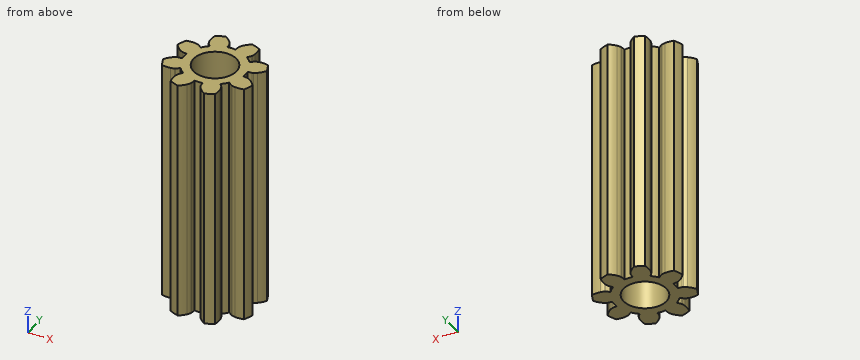
Autodesk Inventor part; units mm, degrees
ref_plane "YZ Plane" through (0, 0, 0) normal (1, 0, 0) x (0, 1, 0)
ref_plane "XZ Plane" through (0, 0, 0) normal (0, 1, 0) x (-1, 0, 0)
ref_plane "XY Plane" through (0, 0, 0) normal (0, 0, 1) x (1, 0, 0)
sketch "Sketch2" plane through (0, 0, 0) normal (0, 0, 1) x (1, 0, 0)
  arc A0 (0.2626, 1.917) -> (0.2462, 1.8632) centre (0.4994, 1.8157) ccw
  arc A1 (0.3627, 2.0876) -> (0.2626, 1.917) centre (0.9307, 1.6395) ccw
  arc A2 (0.7114, 2.3967) -> (0.3627, 2.0876) centre (1.3933, 1.2761) ccw
  arc A3 (-1.1698, 1.5411) -> (-1.1434, 1.4916) centre (-0.9308, 1.637) ccw
  arc A4 (-1.2197, 1.7326) -> (-1.1698, 1.5411) centre (-0.5012, 1.8175) ccw
  arc A5 (-1.1917, 2.1977) -> (-1.2197, 1.7326) centre (0.0829, 1.8876) ccw
  arc A6 (-1.917, 0.2626) -> (-1.8632, 0.2462) centre (-1.8157, 0.4994) ccw
  arc A7 (-2.0876, 0.3627) -> (-1.917, 0.2626) centre (-1.6395, 0.9307) ccw
  arc A8 (-2.3967, 0.7114) -> (-2.0876, 0.3627) centre (-1.2761, 1.3933) ccw
  arc A9 (-1.5411, -1.1698) -> (-1.4916, -1.1434) centre (-1.637, -0.9308) ccw
  arc A10 (-1.7326, -1.2197) -> (-1.5411, -1.1698) centre (-1.8175, -0.5012) ccw
  arc A11 (-2.1977, -1.1917) -> (-1.7326, -1.2197) centre (-1.8876, 0.0829) ccw
  arc A12 (-0.2626, -1.917) -> (-0.2462, -1.8632) centre (-0.4994, -1.8157) ccw
  arc A13 (-0.3627, -2.0876) -> (-0.2626, -1.917) centre (-0.9307, -1.6395) ccw
  arc A14 (-0.7114, -2.3967) -> (-0.3627, -2.0876) centre (-1.3933, -1.2761) ccw
  arc A15 (1.1698, -1.5411) -> (1.1434, -1.4916) centre (0.9308, -1.637) ccw
  arc A16 (1.2197, -1.7326) -> (1.1698, -1.5411) centre (0.5012, -1.8175) ccw
  arc A17 (1.1917, -2.1977) -> (1.2197, -1.7326) centre (-0.0829, -1.8876) ccw
  arc A18 (1.917, -0.2626) -> (1.8632, -0.2462) centre (1.8157, -0.4994) ccw
  arc A19 (2.0876, -0.3627) -> (1.917, -0.2626) centre (1.6395, -0.9307) ccw
  arc A20 (2.3967, -0.7114) -> (2.0876, -0.3627) centre (1.2761, -1.3933) ccw
  arc A21 (1.5411, 1.1698) -> (1.4916, 1.1434) centre (1.637, 0.9308) ccw
  arc A22 (1.7326, 1.2197) -> (1.5411, 1.1698) centre (1.8175, 0.5012) ccw
  arc A23 (2.1977, 1.1917) -> (1.7326, 1.2197) centre (1.8876, -0.0829) ccw
  arc A24 (-0.2462, 1.8632) -> (-0.2626, 1.917) centre (-0.4994, 1.8157) ccw
  arc A25 (-0.2626, 1.917) -> (-0.3627, 2.0876) centre (-0.9307, 1.6395) ccw
  arc A26 (-0.3627, 2.0876) -> (-0.7114, 2.3967) centre (-1.3933, 1.2761) ccw
  arc A27 (-1.4916, 1.1434) -> (-1.5411, 1.1698) centre (-1.637, 0.9308) ccw
  arc A28 (-1.5411, 1.1698) -> (-1.7326, 1.2197) centre (-1.8175, 0.5012) ccw
  arc A29 (-1.7326, 1.2197) -> (-2.1977, 1.1917) centre (-1.8876, -0.0829) ccw
  arc A30 (-1.8632, -0.2462) -> (-1.917, -0.2626) centre (-1.8157, -0.4994) ccw
  arc A31 (-1.917, -0.2626) -> (-2.0876, -0.3627) centre (-1.6395, -0.9307) ccw
  arc A32 (-2.0876, -0.3627) -> (-2.3967, -0.7114) centre (-1.2761, -1.3933) ccw
  arc A33 (-1.1434, -1.4916) -> (-1.1698, -1.5411) centre (-0.9308, -1.637) ccw
  arc A34 (-1.1698, -1.5411) -> (-1.2197, -1.7326) centre (-0.5012, -1.8175) ccw
  arc A35 (-1.2197, -1.7326) -> (-1.1917, -2.1977) centre (0.0829, -1.8876) ccw
  arc A36 (0.2462, -1.8632) -> (0.2626, -1.917) centre (0.4994, -1.8157) ccw
  arc A37 (0.2626, -1.917) -> (0.3627, -2.0876) centre (0.9307, -1.6395) ccw
  arc A38 (0.3627, -2.0876) -> (0.7114, -2.3967) centre (1.3933, -1.2761) ccw
  arc A39 (1.4916, -1.1434) -> (1.5411, -1.1698) centre (1.637, -0.9308) ccw
  arc A40 (1.5411, -1.1698) -> (1.7326, -1.2197) centre (1.8175, -0.5012) ccw
  arc A41 (1.7326, -1.2197) -> (2.1977, -1.1917) centre (1.8876, 0.0829) ccw
  arc A42 (1.8632, 0.2462) -> (1.917, 0.2626) centre (1.8157, 0.4994) ccw
  arc A43 (1.917, 0.2626) -> (2.0876, 0.3627) centre (1.6395, 0.9307) ccw
  arc A44 (2.0876, 0.3627) -> (2.3967, 0.7114) centre (1.2761, 1.3933) ccw
  arc A45 (1.1434, 1.4916) -> (1.1698, 1.5411) centre (0.9308, 1.637) ccw
  arc A46 (1.1698, 1.5411) -> (1.2197, 1.7326) centre (0.5012, 1.8175) ccw
  arc A47 (1.2197, 1.7326) -> (1.1917, 2.1977) centre (-0.0829, 1.8876) ccw
  arc A48 (0.2162, 1.6358) -> (-0.2162, 1.6358) centre (0, 0) ccw
  arc A49 (-1.0038, 1.3095) -> (-1.3095, 1.0038) centre (0, 0) ccw
  arc A50 (-1.6358, 0.2162) -> (-1.6358, -0.2162) centre (0, 0) ccw
  arc A51 (-1.3095, -1.0038) -> (-1.0038, -1.3095) centre (0, 0) ccw
  arc A52 (-0.2162, -1.6358) -> (0.2162, -1.6358) centre (0, 0) ccw
  arc A53 (1.0038, -1.3095) -> (1.3095, -1.0038) centre (0, 0) ccw
  arc A54 (1.6358, -0.2162) -> (1.6358, 0.2162) centre (0, 0) ccw
  arc A55 (1.3095, 1.0038) -> (1.0038, 1.3095) centre (0, 0) ccw
  arc A56 (-0.7114, 2.3967) -> (-1.1917, 2.1977) centre (0, 0) ccw
  arc A57 (-2.1977, 1.1917) -> (-2.3967, 0.7114) centre (0, 0) ccw
  arc A58 (-2.3967, -0.7114) -> (-2.1977, -1.1917) centre (0, 0) ccw
  arc A59 (-1.1917, -2.1977) -> (-0.7114, -2.3967) centre (0, 0) ccw
  arc A60 (0.7114, -2.3967) -> (1.1917, -2.1977) centre (0, 0) ccw
  arc A61 (2.1977, -1.1917) -> (2.3967, -0.7114) centre (0, 0) ccw
  arc A62 (2.3967, 0.7114) -> (2.1977, 1.1917) centre (0, 0) ccw
  arc A63 (1.1917, 2.1977) -> (0.7114, 2.3967) centre (0, 0) ccw
  line L0 (0.2162, 1.6358) -> (0.2462, 1.8632)
  line L1 (-1.0038, 1.3095) -> (-1.1434, 1.4916)
  line L2 (-1.6358, 0.2162) -> (-1.8632, 0.2462)
  line L3 (-1.3095, -1.0038) -> (-1.4916, -1.1434)
  line L4 (-0.2162, -1.6358) -> (-0.2462, -1.8632)
  line L5 (1.0038, -1.3095) -> (1.1434, -1.4916)
  line L6 (1.6358, -0.2162) -> (1.8632, -0.2462)
  line L7 (1.3095, 1.0038) -> (1.4916, 1.1434)
  line L8 (-0.2162, 1.6358) -> (-0.2462, 1.8632)
  line L9 (-1.3095, 1.0038) -> (-1.4916, 1.1434)
  line L10 (-1.6358, -0.2162) -> (-1.8632, -0.2462)
  line L11 (-1.0038, -1.3095) -> (-1.1434, -1.4916)
  line L12 (0.2162, -1.6358) -> (0.2462, -1.8632)
  line L13 (1.3095, -1.0038) -> (1.4916, -1.1434)
  line L14 (1.6358, 0.2162) -> (1.8632, 0.2462)
  line L15 (1.0038, 1.3095) -> (1.1434, 1.4916)
  circle A64 centre (0, 0) radius 1.15
  point P0 (1.3095, 1.0038)
  point P1 (1.0038, 1.3095)
  point P2 (1.1434, 1.4916)
  point P3 (1.1683, 1.5373)
  point P4 (1.2195, 1.7312)
  point P5 (1.1917, 2.1977)
  point P6 (0.7114, 2.3967)
  point P7 (0.3618, 2.0865)
  point P8 (0.261, 1.9131)
  point P9 (0.2462, 1.8632)
  point P10 (0.2162, 1.6358)
  point P11 (-0.2162, 1.6358)
  point P12 (-0.2462, 1.8632)
  point P13 (-0.261, 1.9131)
  point P14 (-0.3618, 2.0865)
  point P15 (-0.7114, 2.3967)
  point P16 (-1.1917, 2.1977)
  point P17 (-1.2195, 1.7312)
  point P18 (-1.1683, 1.5373)
  point P19 (-1.1434, 1.4916)
  point P20 (-1.0038, 1.3095)
  point P21 (-1.3095, 1.0038)
  point P22 (-1.4916, 1.1434)
  point P23 (-1.5373, 1.1683)
  point P24 (-1.7312, 1.2195)
  point P25 (-2.1977, 1.1917)
  point P26 (-2.3967, 0.7114)
  point P27 (-2.0865, 0.3618)
  point P28 (-1.9131, 0.261)
  point P29 (-1.8632, 0.2462)
  point P30 (-1.6358, 0.2162)
  point P31 (-1.6358, -0.2162)
  point P32 (-1.8632, -0.2462)
  point P33 (-1.9131, -0.261)
  point P34 (-2.0865, -0.3618)
  point P35 (-2.3967, -0.7114)
  point P36 (-2.1977, -1.1917)
  point P37 (-1.7312, -1.2195)
  point P38 (-1.5373, -1.1683)
  point P39 (-1.4916, -1.1434)
  point P40 (-1.3095, -1.0038)
  point P41 (-1.0038, -1.3095)
  point P42 (-1.1434, -1.4916)
  point P43 (-1.1683, -1.5373)
  point P44 (-1.2195, -1.7312)
  point P45 (-1.1917, -2.1977)
  point P46 (-0.7114, -2.3967)
  point P47 (-0.3618, -2.0865)
  point P48 (-0.261, -1.9131)
  point P49 (-0.2462, -1.8632)
  point P50 (-0.2162, -1.6358)
  point P51 (0.2162, -1.6358)
  point P52 (0.2462, -1.8632)
  point P53 (0.261, -1.9131)
  point P54 (0.3618, -2.0865)
  point P55 (0.7114, -2.3967)
  point P56 (1.1917, -2.1977)
  point P57 (1.2195, -1.7312)
  point P58 (1.1683, -1.5373)
  point P59 (1.1434, -1.4916)
  point P60 (1.0038, -1.3095)
  point P61 (1.3095, -1.0038)
  point P62 (1.4916, -1.1434)
  point P63 (1.5373, -1.1683)
  point P64 (1.7312, -1.2195)
  point P65 (2.1977, -1.1917)
  point P66 (2.3967, -0.7114)
  point P67 (2.0865, -0.3618)
  point P68 (1.9131, -0.261)
  point P69 (1.8632, -0.2462)
  point P70 (1.6358, -0.2162)
  point P71 (1.6358, 0.2162)
  point P72 (1.8632, 0.2462)
  point P73 (1.9131, 0.261)
  point P74 (2.0865, 0.3618)
  point P75 (2.3967, 0.7114)
  point P76 (2.1977, 1.1917)
  point P77 (1.7312, 1.2195)
  point P78 (1.5373, 1.1683)
  point P79 (1.4916, 1.1434)
  point P80 (1.1698, 1.5411)
  point P81 (1.2197, 1.7326)
  point P82 (0.3627, 2.0876)
  point P83 (0.2626, 1.917)
  point P84 (-0.2626, 1.917)
  point P85 (-0.3627, 2.0876)
  point P86 (-1.2197, 1.7326)
  point P87 (-1.1698, 1.5411)
  point P88 (-1.5411, 1.1698)
  point P89 (-1.7326, 1.2197)
  point P90 (-2.0876, 0.3627)
  point P91 (-1.917, 0.2626)
  point P92 (-1.917, -0.2626)
  point P93 (-2.0876, -0.3627)
  point P94 (-1.7326, -1.2197)
  point P95 (-1.5411, -1.1698)
  point P96 (-1.1698, -1.5411)
  point P97 (-1.2197, -1.7326)
  point P98 (-0.3627, -2.0876)
  point P99 (-0.2626, -1.917)
  point P100 (0.2626, -1.917)
  point P101 (0.3627, -2.0876)
  point P102 (1.2197, -1.7326)
  point P103 (1.1698, -1.5411)
  point P104 (1.5411, -1.1698)
  point P105 (1.7326, -1.2197)
  point P106 (2.0876, -0.3627)
  point P107 (1.917, -0.2626)
  point P108 (1.917, 0.2626)
  point P109 (2.0876, 0.3627)
  point P110 (1.7326, 1.2197)
  point P111 (1.5411, 1.1698)
  dimension "d6" = 2.3
extrude "Extrusion2" add sketch "Sketch2" along normal blind 13
properties part number "ぴにょん" material "Aluminum 2014-T6"
Design review of the part built by this model. Coordinates are the model's own, in mm. Coordinates: 2 decimals unless noted, no trailing zeros. Order: outer loops, then holes, each group sorted by start corner. A loop starts at its lowest first (then second) coordinate and runs counter-clockwise, first axis right, second up. Notation, with made-up numbers: (13, -14.75) -> (20, -14.75) arc R13 cw to (20, -10.75) -> close; hole circle Ø6 at (34.25, 55). An arc over 180 degrees is marked (long way). One line per item, written item: value. Start each with the question number.
Q1. Take a section at A-A, the plane x = 0. State the section outline as (y, z) points, then the cut area to 3 significant figures.
Q2. For probe 1 along Y at (x, z) = (0, 7.5); probe 2 along X at (y, z) = (-1.7, 8.75); probe 3 along Y at (x, z) = (0.85, 1.25), list the stretches that pass through material, from the lowest coordinate up.
Values follow:
1. outline: (-1.65, 0) -> (-1.15, 0) -> (-1.15, 13) -> (-1.65, 13) -> close; (1.15, 0) -> (1.65, 0) -> (1.65, 13) -> (1.15, 13) -> close
1. area: 13.0 mm2
2. probe 1: y = -1.65 to -1.15, 1.15 to 1.65
2. probe 2: x = -1.22 to -0.22, 0.22 to 1.22
2. probe 3: y = -2.35 to -0.77, 0.77 to 2.35
